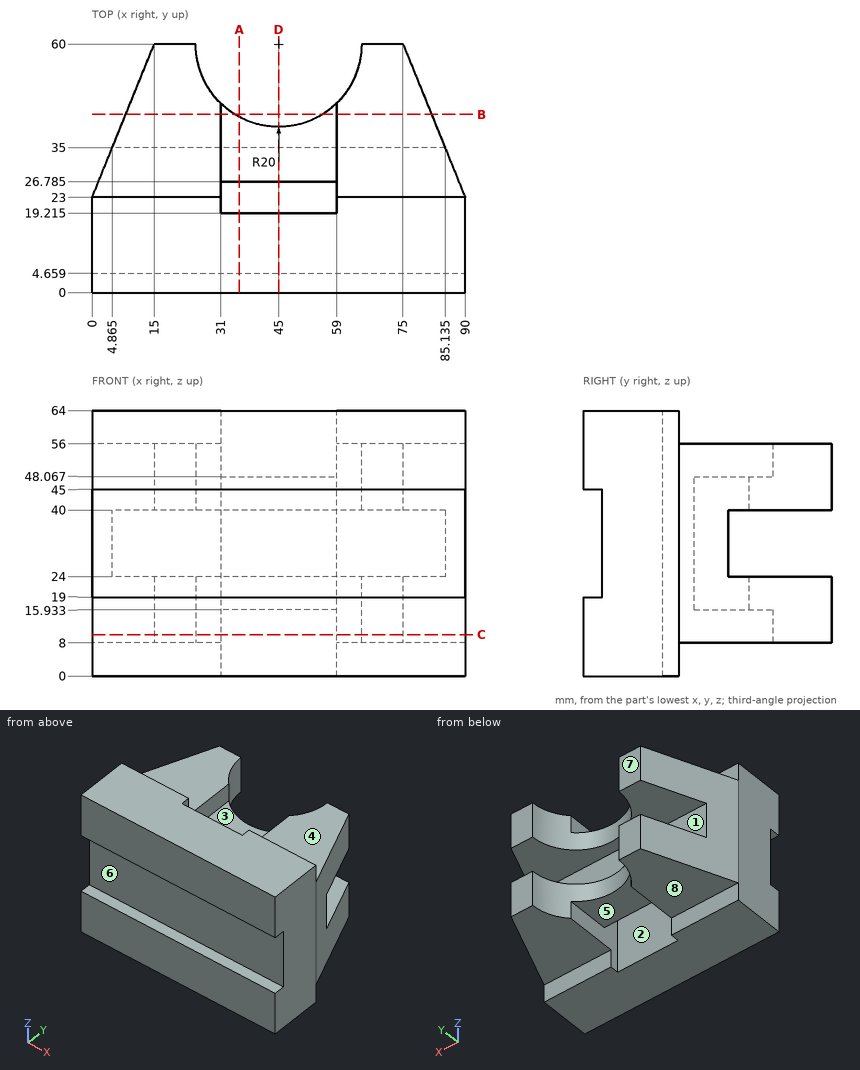
Input: dimensioned drawing with shaded views. Units: mm. Origin: part minimum x, y, z. A direction names the side the tool comes from. Coordinates: 2 decimals unless noted, no trailing zeros. Loops run counter-clockwise (first coordinate to the right, second up) from the corner with the lowest first, then second, coordinate; pieces in that order, holes last. Notation, with made-up numbers: M 81,51 L 137,51 A27 ccw 137,75 Z; hole C 9,72 d5. An arc over 180 degrees is marked long. One line per item, written item: value. Start each with the question number.
1) Draft query along Z for the marked faces 6, 7 and 8. Return one class per face: released by +Z, released by -Z, zero draft, split by the parting line, or undercut.
2) Pin query (flat end, axial travel): P1, Ø15, axis at x = 47.5, y = 35, coming from the -Z side; P2, Ø1.5, axis at x = 21.5, y = 29, coming from the +Z side; P3, Ø14, axis at x = 48, z = 28.5, coming from the -Y side. Return the tip coordinate at first contact, or that it passes through.
3) Cut plane A-A (x = 35.5). Return loops of the section in (y, z) (1 decimal), then the cut area to 3 significant figures.
4) Cut plane D-D (x = 45). Return loops of the section in (y, z) (1 decimal).
5) Material intervals for L1, parallel to Z at x = 26.5, y = 39; L2, parallel to Y at x = 55, z = 33.5 (1 decimal); L3, parallel to Z at x = 74, y = 30, sorted ascending. Write a range as from..to.
6) Cut plane C-C (z = 10). Return loops of the section in (x, y) (1 decimal), then the cut area to 4 significant figures.
7) Reachability of the marked faces 1, 2, 3, 4 and 5 from +Z, -Z, +X, -X, +Y, -Y: full face, straight path, thin tool, end or side. Return the list, or none.
8) Cut plane B-B (y = 43). Return loops of the section in (x, z) (1 decimal).
Evaluation:
1. face 6: undercut
1. face 7: zero draft
1. face 8: released by -Z
2. P1: z = 15.93
2. P2: z = 56
2. P3: y = 4.66
3. outline: M 0,0 L 19.2,0 L 19.2,64 L 0,64 L 0,45 L 4.7,45 L 4.7,19 L 0,19 Z; M 26.8,15.9 L 42.4,15.9 L 42.4,24 L 35,24 L 35,40 L 42.4,40 L 42.4,48.1 L 26.8,48.1 Z
3. area: 1,490 mm^2
4. outline: M 0,0 L 19.2,0 L 19.2,64 L 0,64 L 0,45 L 4.7,45 L 4.7,19 L 0,19 Z; M 26.8,15.9 L 40,15.9 L 40,24 L 35,24 L 35,40 L 40,40 L 40,48.1 L 26.8,48.1 Z
5. L1: 8..24, 40..56
5. L2: 4.7..19.2, 26.8..35
5. L3: 8..56
6. outline: M 0,0 L 90,0 L 90,23 L 75,60 L 65,60 A20 cw 59,45.7 L 59,19.2 L 31,19.2 L 31,45.7 A20 cw 25,60 L 15,60 L 0,23 Z
6. area: 3,585 mm^2
7. face 1: +X, -X, +Y
7. face 2: +Z, -Z
7. face 3: +Z, +Y
7. face 4: +Z, +X, -X, +Y
7. face 5: -Z, +Y
8. outline: M 8.1,8 L 31,8 L 31,15.9 L 34.5,15.9 L 34.5,24 L 8.1,24 Z; M 8.1,40 L 34.5,40 L 34.5,48.1 L 31,48.1 L 31,56 L 8.1,56 Z; M 55.5,15.9 L 59,15.9 L 59,8 L 81.9,8 L 81.9,24 L 55.5,24 Z; M 55.5,40 L 81.9,40 L 81.9,56 L 59,56 L 59,48.1 L 55.5,48.1 Z
